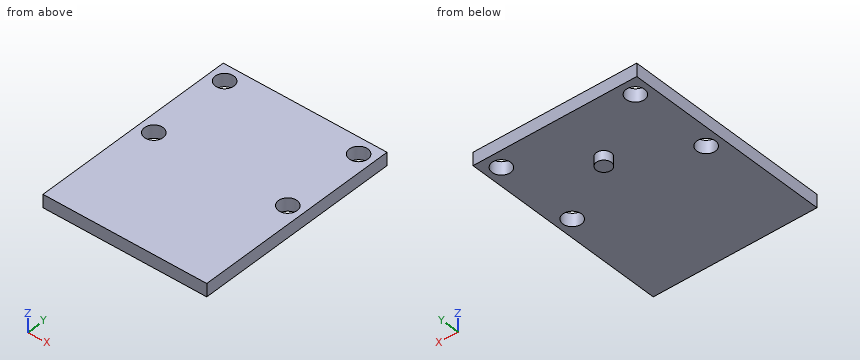
```python
from build123d import *

# Parameters (mm, degrees)
SKETCH1_W           = 22
SKETCH1_H           = 28
SKETCH1_R           = 1.25
BOSS_EXTRUDE1_DEPTH = 1.75
SKETCH2_R           = 1
BOSS_EXTRUDE2_DEPTH = 1.25


with BuildPart() as part:
    # Sketch1 → Boss-Extrude1 (new body)
    with BuildSketch(Plane.XY):
        with Locations((11, 14)):
            Rectangle(SKETCH1_W, SKETCH1_H)
        with Locations((2, 25.9)):
            Circle(SKETCH1_R, mode=Mode.SUBTRACT)
        with Locations((2, 14.9)):
            Circle(SKETCH1_R, mode=Mode.SUBTRACT)
        with Locations((20, 14.9)):
            Circle(SKETCH1_R, mode=Mode.SUBTRACT)
        with Locations((20, 25.9)):
            Circle(SKETCH1_R, mode=Mode.SUBTRACT)
    extrude(amount=BOSS_EXTRUDE1_DEPTH)

    # Sketch2 → Boss-Extrude2 (add)
    with BuildSketch(Plane(origin=(0, 0, 0), x_dir=(-1, 0, 0), z_dir=(0, 0, -1))):
        with Locations(Location((-11, 20.4, 0), (0, 0, 180))):
            Circle(SKETCH2_R)
    extrude(amount=BOSS_EXTRUDE2_DEPTH)


solid = part.part
```
Work out the finished part from the listing and answer in its coordinate system (mm). Give positions to 0.01 mm unless a question says otherwise; leave off trailing zeros. Order: outer loops, then holes, each group sorted by start corner. A loop starts at its lowest first (then second) coordinate and runs counter-clockwise, first axis right, second up.
1. Section A-A, the plane y = 25.9 is taken. Determine the outline of the cut face in (x, z), and give its area (4 significant figures).
Result sheet:
outline: (0, 0) - (0.75, 0) - (0.75, 1.75) - (0, 1.75) - close; (3.25, 0) - (18.75, 0) - (18.75, 1.75) - (3.25, 1.75) - close; (21.25, 0) - (22, 0) - (22, 1.75) - (21.25, 1.75) - close
area: 29.75 mm2
2. Section B-B, the plane x = 20 is taken. Determine the outline of the cut face in (y, z).
Result sheet:
outline: (0, 0) - (13.65, 0) - (13.65, 1.75) - (0, 1.75) - close; (16.15, 0) - (24.65, 0) - (24.65, 1.75) - (16.15, 1.75) - close; (27.15, 0) - (28, 0) - (28, 1.75) - (27.15, 1.75) - close
3. Section C-C, the plane z = 0.4 is taken. Determine the outline of the cut face in (x, y), and give its area (3 significant figures).
Result sheet:
outline: (0, 0) - (22, 0) - (22, 28) - (0, 28) - close; hole circle Ø2.5 at (2, 14.9); hole circle Ø2.5 at (2, 25.9); hole circle Ø2.5 at (20, 14.9); hole circle Ø2.5 at (20, 25.9)
area: 596 mm2
4. Section D-D, the plane x = 11 is taken. Determine the outline of the cut face in (y, z), and give its area (3 significant figures).
Result sheet:
outline: (0, 0) - (19.4, 0) - (19.4, -1.25) - (21.4, -1.25) - (21.4, 0) - (28, 0) - (28, 1.75) - (0, 1.75) - close
area: 51.5 mm2
5. Straight lines are drawn through the part: L1, parallel to Y at x = 20, z = 1; L2, parallel to Z at x = 19.25, y = 10.75. For each, find the intervals that lie inside material, in ascending order.
Result sheet:
L1: y = 0 to 13.65, 16.15 to 24.65, 27.15 to 28
L2: z = 0 to 1.75
6. This flat-tipped pin is pushed along its axis until it touches: P1, Ø3, axis at x = 2, y = 25.9, coming from the -Z side. Where does it stop, or does it pass through?
Result sheet:
P1: stops at z = 0
